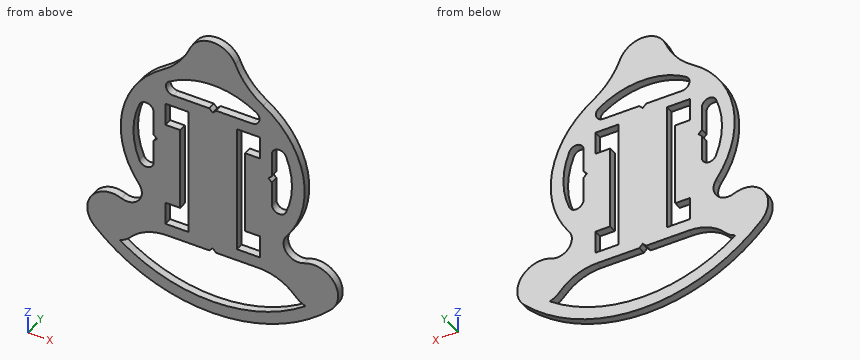
```python
from build123d import *

# Parameters (mm, degrees)
BOSS_EXTRUDE1_DEPTH = 3.175
CUT_EXTRUDE3_REACH  = 5.175
CUT_EXTRUDE4_REACH  = 5.175


with BuildPart() as part:
    # Sketch1 → Boss-Extrude1 (new body)
    with BuildSketch(Plane(origin=(0, 0, 0), x_dir=(1, 0, 0), z_dir=(0, 1, 0))):
        with BuildLine():
            ThreePointArc((-48.171067812, 38.371067812), (0, 58.324177414), (48.171067812, 38.371067812))
            ThreePointArc((48.171067812, 38.371067812), (49.391561976, 25.709830056), (37.196595128, 22.093294269))
            ThreePointArc((37.196595128, 22.093294269), (30.138485199, 20.278544613), (30.037914527, 12.991561861))
            ThreePointArc((30.037914527, 12.991561861), (36.897831444, -16.018932904), (20.532641942, -40.935751303))
            ThreePointArc((20.532641942, -40.935751303), (13.857325378, -46.949439456), (9.262101932, -54.670075305))
            ThreePointArc((9.262101932, -54.670075305), (0, -60.9), (-9.262101932, -54.670075305))
            ThreePointArc((-9.262101932, -54.670075305), (-13.857325378, -46.949439456), (-20.532641942, -40.935751303))
            ThreePointArc((-20.532641942, -40.935751303), (-36.897831444, -16.018932904), (-30.037914527, 12.991561861))
            ThreePointArc((-30.037914527, 12.991561861), (-30.138485199, 20.278544613), (-37.196595128, 22.093294269))
            ThreePointArc((-37.196595128, 22.093294269), (-49.391561976, 25.709830056), (-48.171067812, 38.371067812))
        make_face()
        with BuildLine():
            Line((-18.739320225, 31.3), (18.739320225, 31.3))
            ThreePointArc((18.739320225, 31.3), (26.904286034, 33.042581416), (33.646440075, 37.966666667))
            ThreePointArc((33.646440075, 37.966666667), (35.5534685, 39.620816565), (37.813975674, 40.744683379))
            ThreePointArc((37.813975674, 40.744683379), (0, 53.324177414), (-37.813975674, 40.744683379))
            ThreePointArc((-37.813975674, 40.744683379), (-35.5534685, 39.620816565), (-33.646440075, 37.966666667))
            ThreePointArc((-33.646440075, 37.966666667), (-26.904286034, 33.042581416), (-18.739320225, 31.3))
        make_face(mode=Mode.SUBTRACT)
        with BuildLine():
            Line((-24.1, -20.929751273), (-24.120801343, 1.682420185))
            ThreePointArc((-24.120801343, 1.682420185), (-26.693463619, 4.302078337), (-29.875081258, 2.469454748))
            ThreePointArc((-29.875081258, 2.469454748), (-32.296439432, -9.8), (-29.875081258, -22.069454748))
            ThreePointArc((-29.875081258, -22.069454748), (-26.519157411, -23.87298451), (-24.1, -20.929751273))
        make_face(mode=Mode.SUBTRACT)
        with BuildLine():
            Line((24.1, -20.929751273), (24.1, 1.329751273))
            ThreePointArc((24.1, 1.329751273), (26.519157411, 4.27298451), (29.875081258, 2.469454748))
            ThreePointArc((29.875081258, 2.469454748), (32.296439432, -9.8), (29.875081258, -22.069454748))
            ThreePointArc((29.875081258, -22.069454748), (26.519157411, -23.87298451), (24.1, -20.929751273))
        make_face(mode=Mode.SUBTRACT)
        with BuildLine():
            Line((-16.063354675, -31.3), (16.063354675, -31.3))
            ThreePointArc((16.063354675, -31.3), (18.937942636, -33.441662042), (17.708266649, -36.8088373))
            ThreePointArc((17.708266649, -36.8088373), (0, -42.096439432), (-17.708266649, -36.8088373))
            ThreePointArc((-17.708266649, -36.8088373), (-18.937942636, -33.441662042), (-16.063354675, -31.3))
        make_face(mode=Mode.SUBTRACT)
    extrude(amount=BOSS_EXTRUDE1_DEPTH)

    # Sketch2 → Cut-Extrude3 (cut, up to next)
    with BuildSketch(Plane(origin=(0, 3.175, 0), x_dir=(1, 0, 0), z_dir=(0, 1, 0)), mode=Mode.PRIVATE) as cut_extrude3_sk1:
        Polygon((-19.25, -17.15), (-13.25, -17.15), (-13.25, 17.15), (-19.25, 17.15), (-19.25, 26.45), (-9.95, 26.45), (-9.95, -26.45), (-19.25, -26.45), align=None)
    cut_extrude3_tool1 = extrude(cut_extrude3_sk1.sketch, amount=-CUT_EXTRUDE3_REACH, mode=Mode.PRIVATE) & part.part
    add(cut_extrude3_tool1.solids().sort_by_distance((-16.25, 3.175, 17.687113))[0], mode=Mode.SUBTRACT)
    # Sketch2 → Cut-Extrude3 (cut, up to next)
    with BuildSketch(Plane(origin=(0, 3.175, 0), x_dir=(1, 0, 0), z_dir=(0, 1, 0)), mode=Mode.PRIVATE) as cut_extrude3_sk2:
        Polygon((19.25, -17.15), (13.25, -17.15), (13.25, 17.15), (19.25, 17.15), (19.25, 26.45), (9.95, 26.45), (9.95, -26.45), (19.25, -26.45), align=None)
    cut_extrude3_tool2 = extrude(cut_extrude3_sk2.sketch, amount=-CUT_EXTRUDE3_REACH, mode=Mode.PRIVATE) & part.part
    add(cut_extrude3_tool2.solids().sort_by_distance((16.25, 3.175, 17.687113))[0], mode=Mode.SUBTRACT)

    # Sketch8 → Cut-Extrude4 (cut, up to next)
    with BuildSketch(Plane(origin=(0, 3.175, 0), x_dir=(1, 0, 0), z_dir=(0, 1, 0)), mode=Mode.PRIVATE) as cut_extrude4_sk1:
        Polygon((-22.702010907, -9.63396598), (-24.111696309, -8.21523871), (-24.109105034, -11.032092379), align=None)
    cut_extrude4_tool1 = extrude(cut_extrude4_sk1.sketch, amount=-CUT_EXTRUDE4_REACH, mode=Mode.PRIVATE) & part.part
    add(cut_extrude4_tool1.solids().sort_by_distance((-23.640937, 3.175, 9.627099))[0], mode=Mode.SUBTRACT)
    # Sketch8 → Cut-Extrude4 (cut, up to next)
    with BuildSketch(Plane(origin=(0, 3.175, 0), x_dir=(1, 0, 0), z_dir=(0, 1, 0)), mode=Mode.PRIVATE) as cut_extrude4_sk2:
        Polygon((22.685786438, -9.8), (24.1, -11.214213562), (24.1, -8.385786438), align=None)
    cut_extrude4_tool2 = extrude(cut_extrude4_sk2.sketch, amount=-CUT_EXTRUDE4_REACH, mode=Mode.PRIVATE) & part.part
    add(cut_extrude4_tool2.solids().sort_by_distance((23.628595, 3.175, 9.8))[0], mode=Mode.SUBTRACT)
    # Sketch8 → Cut-Extrude4 (cut, up to next)
    with BuildSketch(Plane(origin=(0, 3.175, 0), x_dir=(1, 0, 0), z_dir=(0, 1, 0)), mode=Mode.PRIVATE) as cut_extrude4_sk3:
        Polygon((0, -29.885786438), (-1.414213562, -31.3), (1.414213562, -31.3), align=None)
    cut_extrude4_tool3 = extrude(cut_extrude4_sk3.sketch, amount=-CUT_EXTRUDE4_REACH, mode=Mode.PRIVATE) & part.part
    add(cut_extrude4_tool3.solids().sort_by_distance((0, 3.175, 30.828595))[0], mode=Mode.SUBTRACT)
    # Sketch8 → Cut-Extrude4 (cut, up to next)
    with BuildSketch(Plane(origin=(0, 3.175, 0), x_dir=(1, 0, 0), z_dir=(0, 1, 0)), mode=Mode.PRIVATE) as cut_extrude4_sk4:
        Polygon((0, 29.885786438), (-1.414213562, 31.3), (1.414213562, 31.3), align=None)
    cut_extrude4_tool4 = extrude(cut_extrude4_sk4.sketch, amount=-CUT_EXTRUDE4_REACH, mode=Mode.PRIVATE) & part.part
    add(cut_extrude4_tool4.solids().sort_by_distance((0, 3.175, -30.828595))[0], mode=Mode.SUBTRACT)


solid = part.part
```
Part model, mm, in its own coordinate system. Coordinates: 2 decimals unless noted, no trailing zeros. Order: outer loops, then holes, each group sorted by start corner. A loop starts at its lowest first (then second) coordinate and runs counter-clockwise, first axis right, second up. Notation, with made-up numbers: (-15.5, 3) -> (20.5, 3) arc R25 ccw to (20.5, 36) -> close; hole circle Ø8 at (-11.75, 16.5). An arc over 180 degrees is marked (long way). Put each result on its own line as item: value. Start each with the question number.
(1) Band-saw the part on B-B (x = -26.5). Give the cut face in (y, z) (3 decimals), then the cut area to 3 significant figures.
(2) Pin check, flat tips, straight feed: pin 1 Ø1.5 at (x, y) = (-13.5, 2) entering from +Z; pin 2 Ø1 at (x, y) = (16.5, 1.5) entering from -Z; pin 3 Ø1 at (x, y) = (10, 1) entering from +Z. Stop position of each tip, or through.
(3) Band-saw the part on D-D (z = 4). Give the cut face in (x, y) (3 decimals), then the cut area to 3 significant figures.
(4) Probe line 1 along Z through (x, y) = (-16.5, 1.3); line 2 along X through (y, z) = (1.8, 15.5) (3 decimals); line 3 along X through (y, z) = (1.3, -12). List the from-to ranges inside material, lowest first. Write a range as [from, to].
(5) Band-saw the part on C-C (z = -47.5). Give the cut face in (x, y) (3 decimals), then the cut area to 3 significant figures.
(6) Band-saw the part on A-A (z = -25). Give the cut face in (x, y) (3 decimals).
Determined:
1. outline: (0, -52.959) -> (3.175, -52.959) -> (3.175, -47.492) -> (0, -47.492) -> close; (0, -32.867) -> (3.175, -32.867) -> (3.175, -4.269) -> (0, -4.269) -> close; (0, 23.869) -> (3.175, 23.869) -> (3.175, 36.056) -> (0, 36.056) -> close
1. area: 147 mm²
2. pin 1: stops at z = 48.39
2. pin 2: stops at z = -56.42
2. pin 3: stops at z = 54.1
3. outline: (-37.07, 0) -> (-31.771, 0) -> (-31.771, 3.175) -> (-37.07, 3.175) -> close; (-24.116, 0) -> (-13.25, 0) -> (-13.25, 3.175) -> (-24.116, 3.175) -> close; (-9.95, 0) -> (9.95, 0) -> (9.95, 3.175) -> (-9.95, 3.175) -> close; (13.25, 0) -> (24.1, 0) -> (24.1, 3.175) -> (13.25, 3.175) -> close; (31.771, 0) -> (37.07, 0) -> (37.07, 3.175) -> (31.771, 3.175) -> close
3. area: 166 mm²
4. line 1: z = [-56.3, -51.13], [-31.3, -26.45], [-17.15, 17.15], [26.45, 31.33], [37.56, 44.12]
4. line 2: x = [-36.986, -31.789], [-24.105, -13.25], [-9.95, 9.95], [13.25, 24.1], [31.789, 36.986]
4. line 3: x = [-30.75, -13.25], [-9.95, 9.95], [13.25, 30.75]
5. outline: (-36.846, 0) -> (-26.483, 0) -> (-26.483, 3.175) -> (-36.846, 3.175) -> close; (26.483, 0) -> (36.846, 0) -> (36.846, 3.175) -> (26.483, 3.175) -> close
5. area: 65.8 mm²
6. outline: (-48.866, 0) -> (-19.25, 0) -> (-19.25, 3.175) -> (-48.866, 3.175) -> close; (-9.95, 0) -> (9.95, 0) -> (9.95, 3.175) -> (-9.95, 3.175) -> close; (19.25, 0) -> (48.866, 0) -> (48.866, 3.175) -> (19.25, 3.175) -> close
